For this review, take the finished solid that the model builds, in its own axes (mm). Face numbers are marked on the shaded views. A direction names the side the tool comes from. Give positions to 0.01 mm unless a question says otherwise; leave off trailing zeros. Write each loop counter-clockwise with the first axis right and the second up, starting at its lowest first coordinate (ties: lowest second). Pieces come first, ordered by that corner, then holes. Notation, with made-up numbers: (-18.5, 68) -> (31.5, 68) arc R13 ccw to (31.5, 89) -> close; hole circle Ø10 at (-1, -2.75). An arc over 180 degrees is marked (long way). Answer as CSV lines item,"result".
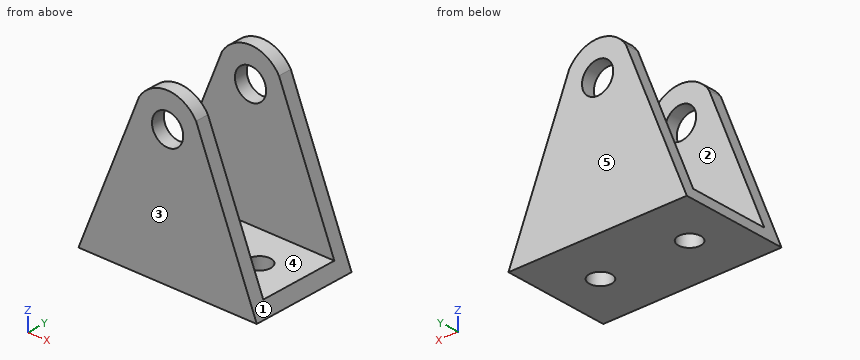
```python
from build123d import *

# Parameters (mm, degrees)
SKETCH_1_R          = 2.5
EXTRUDE_1_DEPTH     = 3
SKETCH_2_W          = 40
SKETCH_2_H          = 3
EXTRUDE_2_DEPTH     = 40
SKETCH_3_R          = 3.5
CUT_EXTRUDE_1_DEPTH = 40


with BuildPart() as part:
    # 草图1 → 凸台-拉伸1 (new body)
    with BuildSketch(Plane.XY):
        Polygon((-29.772681171, 16.394648222), (-29.772681171, -7.605351778), (0.227318829, -7.605351778), (10.227318829, -7.605351778), (10.227318829, 16.394648222), align=None)
        with Locations((-19.772681171, 4.394648222)):
            Circle(SKETCH_1_R, mode=Mode.SUBTRACT)
        with Locations((0.227318829, 4.394648222)):
            Circle(SKETCH_1_R, mode=Mode.SUBTRACT)
    extrude(amount=EXTRUDE_1_DEPTH)

    # 草图2 → 凸台-拉伸2 (add)
    with BuildSketch(Plane.XY.offset(3)):
        with Locations((-9.772681171, -6.105351778)):
            Rectangle(SKETCH_2_W, SKETCH_2_H)
        with Locations((-9.772681171, 14.894648222)):
            Rectangle(SKETCH_2_W, SKETCH_2_H)
    extrude(amount=EXTRUDE_2_DEPTH)

    # 草图3 → 切除-拉伸1 (cut)
    with BuildSketch(Plane.XZ.offset(7.605351778)):
        with Locations((-9.772681171, 30)):
            Circle(SKETCH_3_R)
        with BuildLine():
            Line((-29.772681171, 0), (-66.242845542, 33.938537382))
            Line((-66.242845542, 33.938537382), (4.749976108, 60.991202945))
            Line((4.749976108, 60.991202945), (36.387923144, 40.281675758))
            Line((36.387923144, 40.281675758), (10.227318829, 0))
            Line((10.227318829, 0), (-3.390054495, 33.938537382))
            ThreePointArc((-3.390054495, 33.938537382), (-9.772681171, 37.5), (-16.155307848, 33.938537382))
            Line((-16.155307848, 33.938537382), (-29.772681171, 0))
        make_face()
    extrude(amount=-CUT_EXTRUDE_1_DEPTH, mode=Mode.SUBTRACT)


solid = part.part
```
Q1. Add section A-A (y = 3.25). Write out the cut boundary in (x, z).
Answer block:
outline,"(-29.77, 0) -> (-22, 0) -> (-22, 3) -> (-28.57, 3) -> close; (-17.55, 0) -> (-2, 0) -> (-2, 3) -> (-17.55, 3) -> close; (2.45, 0) -> (10.23, 0) -> (9.02, 3) -> (2.45, 3) -> close"
Q2. For the marked faces 4 and 5, list the 3-axis set-ups (+Z, -Z, +X, -X, +Y, -Y) from which the entire face can be reached by the end or side of a thin tool; tool diameter is ignored.
Answer block:
face 4,"+Z, +X, -X"
face 5,"+Z, -Z, +X, -X, +Y"
Q3. Add section D-D (z = 30). Write out the cut boundary in (x, y), plus the area to 3 significant figures.
Answer block:
outline,"(-17.74, -7.61) -> (-13.27, -7.61) -> (-13.27, -4.61) -> (-17.74, -4.61) -> close; (-17.74, 13.39) -> (-13.27, 13.39) -> (-13.27, 16.39) -> (-17.74, 16.39) -> close; (-6.27, -7.61) -> (-1.81, -7.61) -> (-1.81, -4.61) -> (-6.27, -4.61) -> close; (-6.27, 13.39) -> (-1.81, 13.39) -> (-1.81, 16.39) -> (-6.27, 16.39) -> close"
area,"53.6 mm2"
Q4. Draft analysis for pull direction Y (two halves, no side actions). For the marked faces 1, 2 and 3, state which applies: released by +Y, released by -Y, zero draft, split by the parting line, or undercut.
Answer block:
face 1,"zero draft"
face 2,"undercut"
face 3,"released by -Y"
Q5. Clearance check with flat-ended pins moving along their axes: pin 1 (4 mm diameter, centred on x = -9.77, z = 30, fed in from -Y); pin 2 (8 mm diameter, centred on y = 13.5, z = 33.5, fed in from -X); pin 3 (5 mm diameter, centred on x = -6, y = 11.5, fed in from +Z). State where each tip first meets the part, or that it passes through.
Answer block:
pin 1,"passes through"
pin 2,"stops at x = -17.94"
pin 3,"stops at z = 37.19"
Q6. Add section C-C (z = 14). Write out the cut boundary in (x, y).
Answer block:
outline,"(-24.16, -7.61) -> (4.61, -7.61) -> (4.61, -4.61) -> (-24.16, -4.61) -> close; (-24.16, 13.39) -> (4.61, 13.39) -> (4.61, 16.39) -> (-24.16, 16.39) -> close"
Q7. Add section B-B (x = -19). Write out the cut boundary in (y, z), plus the area to 3 significant figures.
Answer block:
outline,"(-7.61, 0) -> (2.02, 0) -> (2.02, 3) -> (-4.61, 3) -> (-4.61, 26.85) -> (-7.61, 26.85) -> close; (6.77, 0) -> (16.39, 0) -> (16.39, 26.85) -> (13.39, 26.85) -> (13.39, 3) -> (6.77, 3) -> close"
area,"201 mm2"
Q8. To check wall thickness, follow probe 1 along Y at (x, z) = (-4.5, 4.5); probe 2 along Z at (x, y) = (-24, 7); probe 3 along Z at (x, y) = (-9, 14.5). State the ranges of each line that lie inside material, in increasing order. Write a range as [from, to].
Answer block:
probe 1,"y = [-7.61, -4.61], [13.39, 16.39]"
probe 2,"z = [0, 3]"
probe 3,"z = [0, 26.59], [33.41, 37.46]"
